Part print with two shaded views. Sizes in mm from the minimum x, y, z corner. A direction names the side the tool comes from. Give positions to 0.01 mm unless a question says otherwise; leave off trailing zeros. Write each loop counter-clockwise with the first axis right and the second up, starting at its lowest first coordinate (ties: lowest second). Pieces come first, ordered by that corner, then holes.
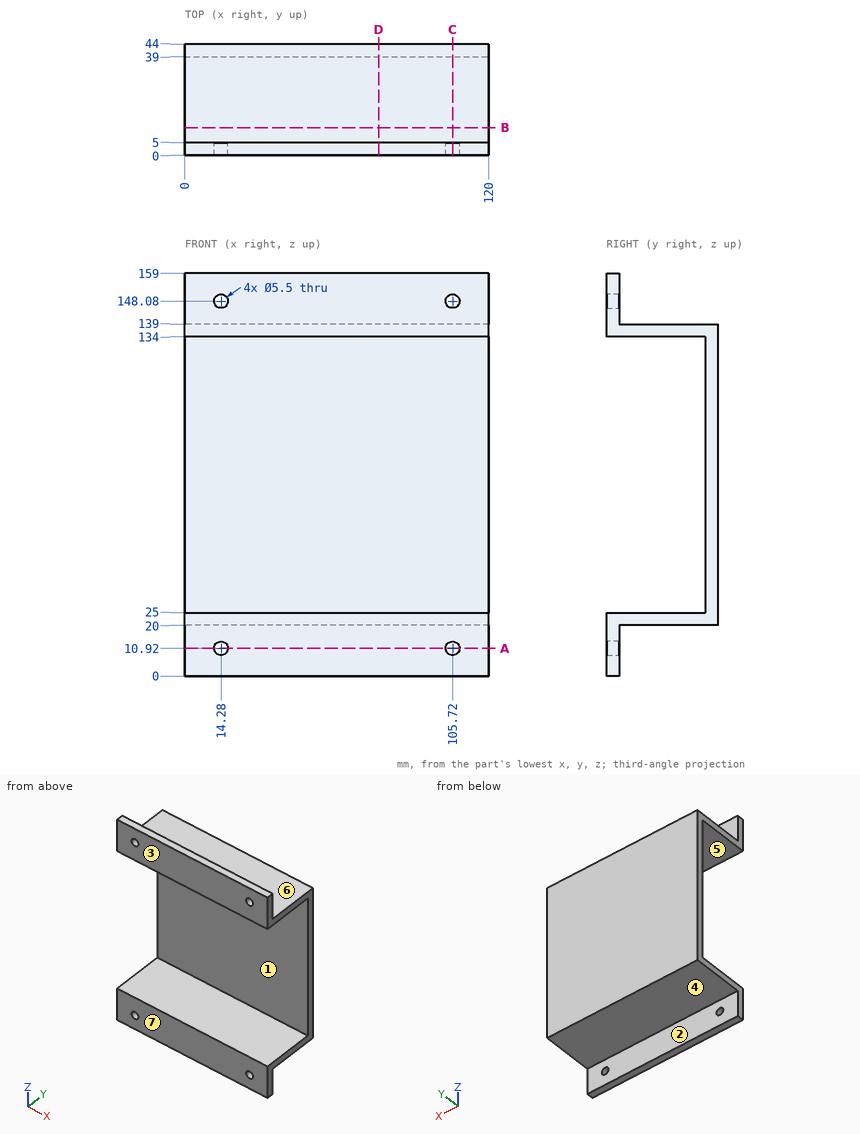
1) Saw through at B-B (y = 11). Write the cut outline in (x, z), and give its area (3 significant figures).
Check result:
outline: (0, 20) - (120, 20) - (120, 25) - (0, 25) - close; (0, 134) - (120, 134) - (120, 139) - (0, 139) - close
area: 1,200 mm2
2) Saw through at C-C (x = 105.72). Write the cut outline in (y, z), and give its area (3 significant figures).
Check result:
outline: (0, 0) - (5, 0) - (5, 8.17) - (0, 8.17) - close; (0, 13.67) - (5, 13.67) - (5, 20) - (44, 20) - (44, 139) - (5, 139) - (5, 145.33) - (0, 145.33) - (0, 134) - (39, 134) - (39, 25) - (0, 25) - close; (0, 150.83) - (5, 150.83) - (5, 159) - (0, 159) - close
area: 1,130 mm2
3) Drill centre lines: L1, parallel to X at y = 2.6, z = 10.92; L2, parallel to Z at x = 105.72, y = 1.3; L3, parallel to Z at x = 35.5, y = 8. Where is each one in solid material? Low to high.
Check result:
L1: x = 0 to 11.53, 17.03 to 102.97, 108.47 to 120
L2: z = 0 to 8.17, 13.67 to 25, 134 to 145.33, 150.83 to 159
L3: z = 20 to 25, 134 to 139
4) Mould opens along Z. For the marked faces 4, 5, 6 and 7 say: +Z half, -Z half, draft (parallel to the pull), parting line (faces both ways), or undercut.
Check result:
face 4: -Z half
face 5: undercut
face 6: +Z half
face 7: draft
5) Saw through at A-A (z = 10.92). Write the cut outline in (x, y).
Check result:
outline: (0, 0) - (11.53, 0) - (11.53, 5) - (0, 5) - close; (17.03, 0) - (102.97, 0) - (102.97, 5) - (17.03, 5) - close; (108.47, 0) - (120, 0) - (120, 5) - (108.47, 5) - close
6) 3-axis set-ups, long thin cutter, end or side, ignore diameter. For the marked faces 1, 2 and 3: which of +Z, -Z, +X, -X, +Y, -Y reach the whole face in a straight line?
Check result:
face 1: +X, -X, -Y
face 2: -Z, +X, -X, +Y
face 3: +Z, -Z, +X, -X, -Y
7) Saw through at D-D (x = 76.5). Write the cut outline in (y, z).
Check result:
outline: (0, 0) - (5, 0) - (5, 20) - (44, 20) - (44, 139) - (5, 139) - (5, 159) - (0, 159) - (0, 134) - (39, 134) - (39, 25) - (0, 25) - close
8) Flat gauge pins, fed straight in: P1, Ø22, axis at x = 56, z = 152.5, coming from the +Y side; P2, Ø10, axis at x = 64, z = 126, coming from the -Y side; P3, Ø12, axis at x = 71.5, y = 17.5, coming from the +Z side; P4, Ø4.5, axis at x = 14.28, z = 148.08, coming from the -Y side. Where does each tip first touch, or does it go through?
Check result:
P1: stops at y = 5
P2: stops at y = 39
P3: stops at z = 139
P4: passes through
